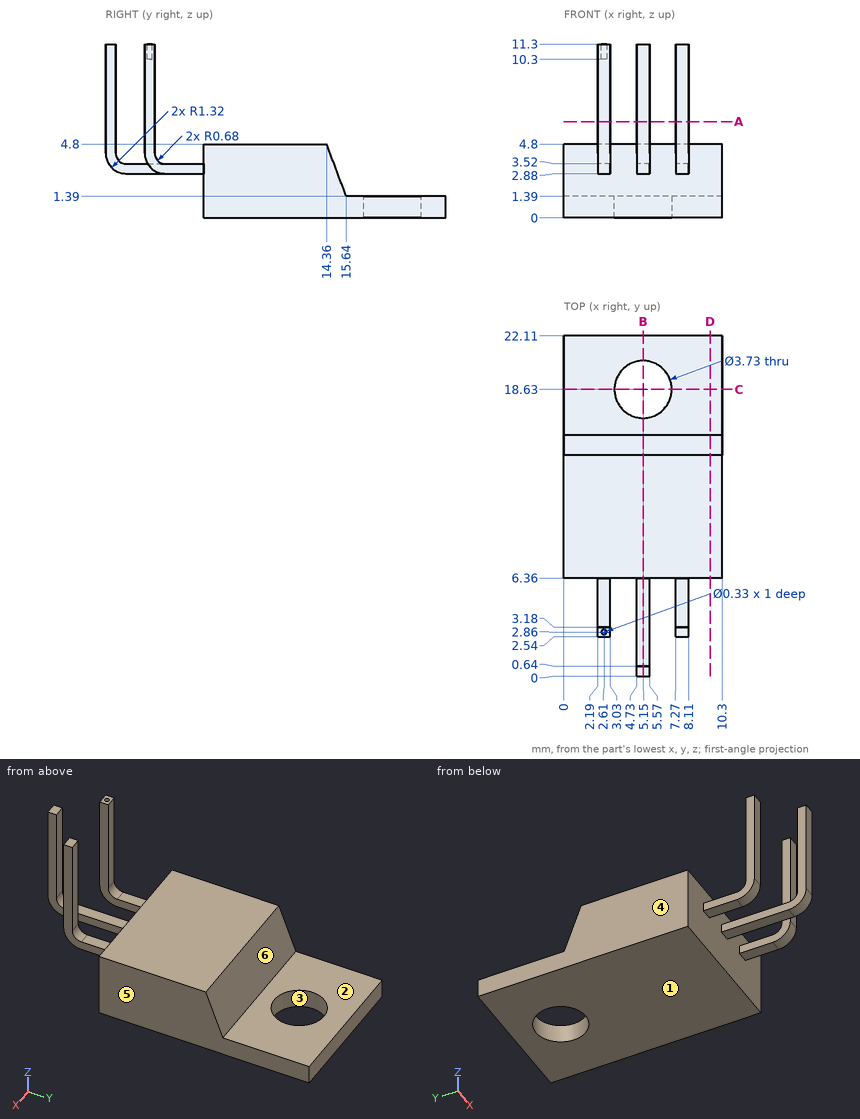
Answer from the drawing. Dimensions are ordinates in mm from the lowest x, y and z of the part. A direction names the side the tool comes from. Coordinates: 2 decimals unless noted, no trailing zeros. Order: outer loops, then holes, each group sorted by start corner. A loop starts at its lowest first (then second) coordinate and runs counter-clockwise, first axis right, second up. Notation, with made-up numbers: (-9.5, -14) - (10.5, -14) arc R14 ccw to (10.5, 11) - close; hole circle Ø3 at (-25, -12.5). An arc over 180 degrees is marked (long way). Put each result on its own line as item: value. Start each with the question number.
1) Find section A-A (z = 6.25). Give the vertices of the cut face in (x, y).
2) For the marked faces 1 and 2, determine the directions among +Z, -Z, +X, -X, +Y, -Y from which every point of the face is accessible in a straight line to the end or side of a thin tool.
3) Find section D-D (x = 9.5). Give the vertices of the cut face in (y, z).
4) Flat-ended cylindrical pins translate along their axes: pin 1 (3 mm diameter, centred on y = 4.5, z = 9, fed in from -X); pin 2 (1.5 mm diameter, centred on x = 5, z = 3.5, fed in from +Y); pin 3 (2.5 mm diameter, centred on x = 3.5, y = 12, fed in from +Z); pin 4 (1 mm diameter, centred on y = 10, z = 6, fed in from -X). Find the tip coordinate at first contact, or state that the pin passes through.
5) Find the intervals of material crossed by line 1 (Y direction, x = 5.15, z = 0.45) (1 decimal); line 2 (Y direction, x = 5.25, z = 5.5); line 3 (Y direction, x = 2.61, z = 10.95) (1 decimal), in increasing order. Write a range as from..to.
6) Find section B-B (x = 5.15). Give the vertices of the cut face in (y, z) (1 decimal).
7) Find section C-C (y = 18.63). Give the vertices of the cut face in (x, z) (1 decimal).
8) For a pull along X with two mould halves and no side action, classify the marked faces 3, 4, 5 and 6 as released by +X, released by -X, zero draft, split by the parting line, or undercut.
Results list:
1. outline: (2.19, 2.54) - (3.03, 2.54) - (3.03, 3.18) - (2.19, 3.18) - close; (4.73, 0) - (5.57, 0) - (5.57, 0.64) - (4.73, 0.64) - close; (7.27, 2.54) - (8.11, 2.54) - (8.11, 3.18) - (7.27, 3.18) - close
2. face 1: -Z, +X, -X, +Y, -Y
2. face 2: +Z, +X, -X, +Y
3. outline: (6.36, 0) - (22.11, 0) - (22.11, 1.39) - (15.64, 1.39) - (14.36, 4.8) - (6.36, 4.8) - close
4. pin 1: stops at x = 2.19
4. pin 2: stops at y = 15.13
4. pin 3: stops at z = 4.8
4. pin 4: passes through
5. line 1: y = 6.4..16.8, 20.5..22.1
5. line 2: y = 0..0.64
5. line 3: y = 2.5..2.7, 3..3.2
6. outline: (0, 4.2) arc R1.3 ccw to (1.3, 2.9) - (6.4, 2.9) - (6.4, 0) - (16.8, 0) - (16.8, 1.4) - (15.6, 1.4) - (14.4, 4.8) - (6.4, 4.8) - (6.4, 3.5) - (1.3, 3.5) arc R0.7 cw to (0.6, 4.2) - (0.6, 11.3) - (0, 11.3) - close; (20.5, 0) - (22.1, 0) - (22.1, 1.4) - (20.5, 1.4) - close
7. outline: (0, 0) - (3.3, 0) - (3.3, 1.4) - (0, 1.4) - close; (7, 0) - (10.3, 0) - (10.3, 1.4) - (7, 1.4) - close
8. face 3: undercut
8. face 4: released by -X
8. face 5: released by +X
8. face 6: zero draft
